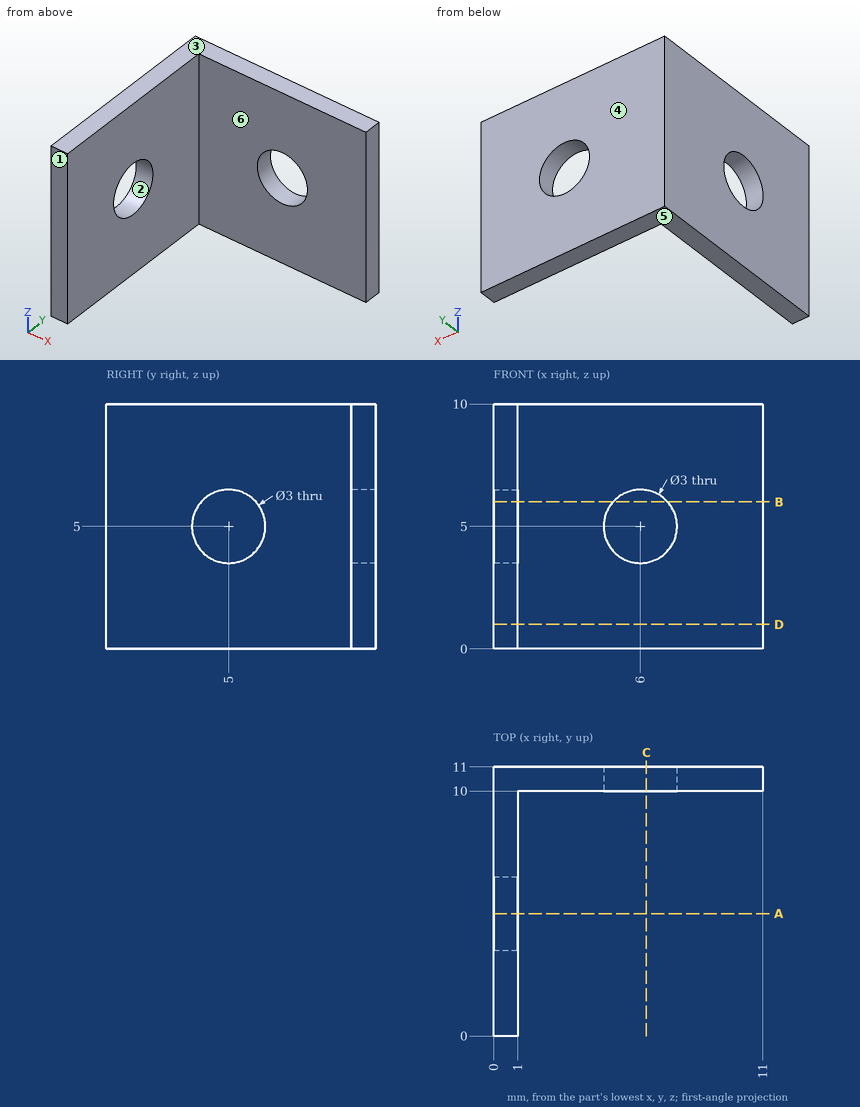
Part print with two shaded views. Sizes in mm from the minimum x, y, z corner. A direction names the side the tool comes from. Give positions to 0.01 mm unless a question says otherwise; leave off trailing zeros. Order: outer loops, then holes, each group sorted by start corner. A loop starts at its lowest first (then second) coordinate and runs counter-clockwise, first axis right, second up. Notation, with made-up numbers: M 52,-4.5 L 74,-4.5 A19 ccw 74,22.5 Z; hole C 35,89 d11. An arc over 180 degrees is marked long. Write item = value, one per line.
Q1. Tool access for the marked faces 5 and 6: list every direction of +Z, -Z, +X, -X, +Y, -Y with a clear straight run to the whole face (end or side of a thin tool).
Derived:
face_5 = -Z, +X, -X, +Y, -Y
face_6 = +Z, -Z, +X, -Y
Q2. Flat gauge pins, fed straight in: pin 1 (2 mm diameter, centred on x = 3, y = 4, fed in from -Z); pin 2 (3 mm diameter, centred on x = 5.5, z = 3, fed in from -Y); pin 3 (1 mm diameter, centred on y = 4, z = 7.5, fed in from +X). Where does each tip first touch, or does it go through?
Derived:
pin_1 = through
pin_2 = 10
pin_3 = 1
Q3. Drill centre lines: line 1 (Z direction, x = 6, y = 10.3); line 2 (Y direction, x = 0.6, z = 5); line 3 (Y direction, x = 3.5, z = 4.5). Where is each one in solid material? Low to high. Write a range as [from, to].
Derived:
line_1 = [0, 3.5], [6.5, 10]
line_2 = [0, 3.5], [6.5, 11]
line_3 = [10, 11]
Q4. Cut at D-D, the plane z = 1. List the corners of the cut face in (x, y).
Derived:
outline = M 0,0 L 1,0 L 1,10 L 11,10 L 11,11 L 0,11 Z
Q5. Cut at A-A, the plane y = 5. List the corners of the cut face in (x, z), then the cut area to 3 significant figures.
Derived:
outline = M 0,0 L 1,0 L 1,3.5 L 0,3.5 Z; M 0,6.5 L 1,6.5 L 1,10 L 0,10 Z
area = 7.00 mm2
Q6. Cut at C-C, the plane x = 6.25. List the corners of the cut face in (y, z), then the cut area to 3 significant figures.
Derived:
outline = M 10,0 L 11,0 L 11,3.52 L 10,3.52 Z; M 10,6.48 L 11,6.48 L 11,10 L 10,10 Z
area = 7.04 mm2
Q7. Two-plate mould, pull along Y, no slides. Class the marked faces 1, 2, 3 and 4: pulls with the +Y half, pulls with the -Y half, needs draft (parallel to the pull), parting line crosses it, or undercut.
Derived:
face_1 = pulls with the -Y half
face_2 = undercut
face_3 = needs draft
face_4 = pulls with the +Y half
Q8. Cut at B-B, the plane z = 6. List the corners of the cut face in (x, y), then the cut area to 3 significant figures.
Derived:
outline = M 0,0 L 1,0 L 1,3.88 L 0,3.88 Z; M 0,6.12 L 1,6.12 L 1,10 L 4.88,10 L 4.88,11 L 0,11 Z; M 7.12,10 L 11,10 L 11,11 L 7.12,11 Z
area = 16.5 mm2
